Design review of the part built by this model. Coordinates are the model's own, in mm. Face numbers are marked on the shaded views. A direction names the side the tool comes from. Coordinates: 2 decimals unless noted, no trailing zeros. Order: outer loops, then holes, each group sorted by start corner. A loop starts at its lowest first (then second) coordinate and runs counter-clockwise, first axis right, second up. Notation, with made-up numbers: M 47,29.25 L 99,29.25 A24 cw 99,49.25 Z; hole C 77.5,9.25 d9. An arc over 180 degrees is marked long. Answer as a JSON object with one key per item and string values.
from build123d import *

# Parameters (mm, degrees)
BOSS_EXTRUDE1_DEPTH = 7.5
CUT_EXTRUDE6_DEPTH  = 5
BOSS_EXTRUDE2_START = -20
BOSS_EXTRUDE2_DEPTH = 5
CHAMFER1_SIZE       = 2
SKETCH11_W          = 14.8
SKETCH11_H          = 9.8
SKETCH11_W_2        = 6.2
SKETCH11_H_2        = 2.8
BOSS_EXTRUDE3_DEPTH = 4.8


with BuildPart() as part:
    # Sketch1 → Boss-Extrude1 (new body)
    with BuildSketch(Plane(origin=(0, 0, 0), x_dir=(1, 0, 0), z_dir=(0, 1, 0))):
        with BuildLine():
            Line((0, 0), (0, 15))
            Line((0, 15), (16, 15))
            ThreePointArc((16, 15), (23.071067812, 17.928932188), (26, 25))
            Line((26, 25), (26, 115))
            Line((26, 115), (41, 115))
            Line((41, 115), (41, 25))
            ThreePointArc((41, 25), (43.928932188, 17.928932188), (51, 15))
            Line((51, 15), (67, 15))
            Line((67, 15), (67, 0))
            Line((67, 0), (0, 0))
        make_face()
    extrude(amount=BOSS_EXTRUDE1_DEPTH)

    # Cut-Sweep1: sweep along a path in Sketch2
    with BuildLine(Plane(origin=(0, 7.5, 0), x_dir=(1, 0, 0), z_dir=(0, 1, 0))) as cut_sweep1_path:
        Line((33.5, 115), (33.5, 7.5))
        Line((33.5, 7.5), (67, 7.5))
    # Sketch3 → Cut-Sweep1 (sweep, cut)
    with BuildSketch(Plane(origin=(0, 0, -115), x_dir=(-1, 0, 0), z_dir=(0, 0, -1))):
        Polygon((-37.6, 5.132863896), (-33.5, 2.765727793), (-29.4, 5.132863896), (-29.4, 9.867136104), (-33.5, 12.234272207), (-37.6, 9.867136104), align=None)
    sweep(path=cut_sweep1_path.line, transition=Transition.RIGHT, mode=Mode.SUBTRACT)

    # Sketch7 → Cut-Extrude6 (cut)
    with BuildSketch(Plane(origin=(0, 7.5, 0), x_dir=(1, 0, 0), z_dir=(0, 1, 0))):
        with BuildLine():
            Line((47.6, 11.6), (47.6, 3.4))
            Line((47.6, 3.4), (29.4, 3.4))
            Line((29.4, 3.4), (29.4, 21.6))
            Line((29.4, 21.6), (37.6, 21.6))
            Line((37.6, 21.6), (37.6, 20.6))
            ThreePointArc((37.6, 20.6), (40.236038969, 14.236038969), (46.6, 11.6))
            Line((46.6, 11.6), (47.6, 11.6))
        make_face()
    extrude(amount=-CUT_EXTRUDE6_DEPTH, mode=Mode.SUBTRACT)

    # Sketch10 → Boss-Extrude2 (add)
    with BuildSketch(Plane(origin=(0, 0, -115), x_dir=(-1, 0, 0), z_dir=(0, 0, -1)).offset(BOSS_EXTRUDE2_START)):
        Polygon((-41, 7.5), (-46, 7.5), (-46, -5), (-21, -5), (-21, 7.5), (-26, 7.5), (-26, 0), (-41, 0), align=None)
    extrude(amount=-BOSS_EXTRUDE2_DEPTH)

    # Chamfer1
    chamfer1_edges = [part.edges().sort_by_distance(p)[0] for p in [
        (26, 0, -57.5),
        (41, 0, -105),
        (33.5, 0, 0),
        (8, 0, -15),
        (23.071067812, 0, -17.928932188),
        (26, 0, -105),
        (41, 0, -57.5),
        (43.928932188, 0, -17.928932188),
        (59, 0, -15),
    ]]
    chamfer(chamfer1_edges, length=CHAMFER1_SIZE)

    # Sketch11 → Boss-Extrude3 (add)
    with BuildSketch(Plane(origin=(0, 7.5, 0), x_dir=(1, 0, 0), z_dir=(0, 1, 0))):
        with Locations((12.5, 7.5)):
            Rectangle(SKETCH11_W, SKETCH11_H)
        with Locations((25.2, 92.5)):
            Rectangle(SKETCH11_W_2, SKETCH11_H_2)
        with Locations((41.8, 92.5)):
            Rectangle(SKETCH11_W_2, SKETCH11_H_2)
    extrude(amount=BOSS_EXTRUDE3_DEPTH)


with BuildPart() as body_2:
    # Mirror1: mirrored copy
    add(part.part.mirror(Plane.ZX.offset(7.5)))


solid = body_2.part
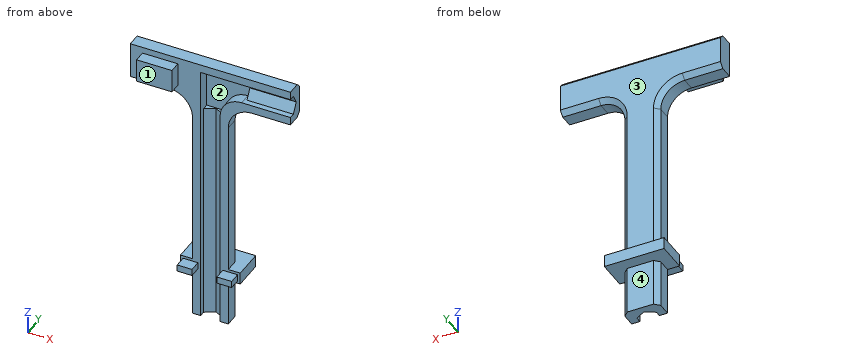
1) Mouldability with a two-part tool opening along Z and no side actions: class the marked faces 1 and 2 as released by +Z, released by -Z, zero draft, split by the parting line, or undercut.
Taken from the geometry:
{"face 1": "zero draft", "face 2": "undercut"}
2) Insertion check: pin 1 Ø3 at (y, z) = (10, -65) entering from +X; pin 2 Ø1.4 at (y, z) = (4, -92) entering from -X; pin 3 Ø4 at (x, y) = (15, 5) entering from +Z; pin 4 Ø2 at (y, z) = (5, -79.5) entering from +X. Each pin has a flat end and moves straight along its axis. Give the tip position at first contact, or say it passes through.
Taken from the geometry:
{"pin 1": "stops at x = 41", "pin 2": "stops at x = 22.1", "pin 3": "stops at z = -2.6", "pin 4": "passes through"}
3) To check wall thickness, follow L1, parallel to X at y = 8.75, z = -96; L2, parallel to Y at x = 37, z = -16.5; L3, parallel to Z at x = 5, y = 12.5. State the ranges of each line that lie inside material, in increasing order.
Taken from the geometry:
{"L1": "x = 26 to 29.4, 37.6 to 41", "L2": "y = 12.5 to 15", "L3": "z = -15 to 0"}
4) Add section D-D (x = 53). State the section outline as (y, z) points.
Taken from the geometry:
{"outline": "M 7.5,-15 L 13,-15 L 15,-13 L 15,-2 L 13,0 L 7.5,0 L 7.5,-3.4 L 9.87,-3.4 L 12.23,-7.5 L 9.87,-11.6 L 7.5,-11.6 Z"}
5) Add section C-C (z = -65.5). State the section outline as (x, y) points, and give its area (3 significant figures).
Taken from the geometry:
{"outline": "M 26,7.5 L 29.4,7.5 L 29.4,9.87 L 33.5,12.23 L 37.6,9.87 L 37.6,7.5 L 41,7.5 L 41,13 L 39,15 L 28,15 L 26,13 Z", "area": "79.4 mm2"}
6) Add section B-B (x = 9). State the section outline as (y, z) points, and give its area (3 significant figures).
Taken from the geometry:
{"outline": "M 2.7,-12.4 L 7.5,-12.4 L 7.5,-15 L 13,-15 L 15,-13 L 15,-2 L 13,0 L 7.5,0 L 7.5,-2.6 L 2.7,-2.6 Z", "area": "156 mm2"}
7) Tool access review of the marked faces 3 and 4: name each direction out of +Z, -Z, +X, -X, +Y, -Y from which nothing blocks a thin tool from reaching the whole face with its end or side.
Taken from the geometry:
{"face 3": "+Z, +X, -X, +Y", "face 4": "-Z, +X, -X, +Y"}
8) Add section A-A (y = 5.75). State the section outline as (x, z) points.
Taken from the geometry:
{"outline": "M 5.1,-12.4 L 19.9,-12.4 L 19.9,-2.6 L 5.1,-2.6 Z; M 22.1,-93.9 L 28.3,-93.9 L 28.3,-91.1 L 22.1,-91.1 Z; M 38.7,-93.9 L 44.9,-93.9 L 44.9,-91.1 L 38.7,-91.1 Z"}
